The drawing under review shows one solid part. Ordinate dimensions are in mm from its lowest x, y, z. A direction names the side the tool comes from. Round coordinates to 2 decimals unless told otherwise and drop trailing zeros. Order: outer loops, then holes, each group sorted by start corner. A loop starts at its lowest first (then second) coordinate and runs counter-clockwise, first axis right, second up. Notation, with made-up numbers: M 63.5,-23 L 91.5,-23 A35 ccw 91.5,11 Z; hole C -4,29.5 d7. An arc over 180 degrees is marked long. Write item = value, one per line. Start each with the question number.
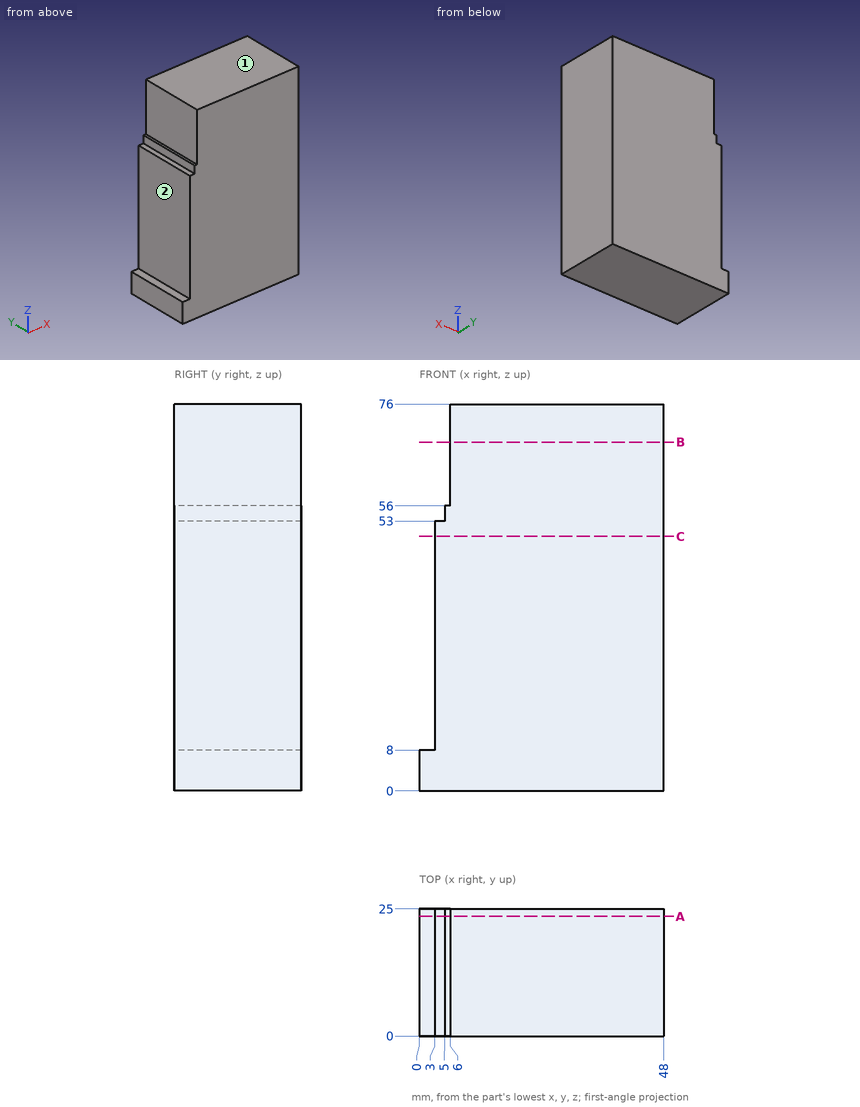
(1) Consider section C-C, the plane z = 50. Write out the cut boundary in (x, y), then the cut area to 4 significant figures.
(2) For line 1 along X through (y, z) = (16.5, 40); line 2 along X through (y, z) = (5.75, 65), list the stretches that pass through material, from the lowest coordinate up. Write a range as [from, to].
(3) Consider section A-A, the plane y = 23.5. Write out the cut boundary in (x, z).
(4) Consider section B-B, the plane z = 68.5. Write out the cut boundary in (x, y), then the cut area to 3 significant figures.
(5) For the marked faces 1 and 2, list the 3-axis set-ups (+Z, -Z, +X, -X, +Y, -Y) from which the entire face can be reached by the end or side of a thin tool; tool diameter is ignored.
(6) Insertion check: pin 1 (12 mm diameter, centred on y = 15, z = 15.5, fed in from -X); pin 2 (0.8 mm diameter, centred on x = 5.5, y = 17.5, fed in from +Z); pin 3 (2.5 mm diameter, centred on y = 7, z = 55, fed in from -X). Each pin has a flat end and moves straight along its axis. Give the tip position at first contact, or say it passes through.
Completed:
q1.outline = M 3,0 L 48,0 L 48,25 L 3,25 Z
q1.area = 1,125 mm2
q2.line_1 = [3, 48]
q2.line_2 = [6, 48]
q3.outline = M 0,0 L 48,0 L 48,76 L 6,76 L 6,56 L 5,56 L 5,53 L 3,53 L 3,8 L 0,8 Z
q4.outline = M 6,0 L 48,0 L 48,25 L 6,25 Z
q4.area = 1,050 mm2
q5.face_1 = +Z, +X, -X, +Y, -Y
q5.face_2 = +Z, -X, +Y, -Y
q6.pin_1 = 3
q6.pin_2 = 56
q6.pin_3 = 5
